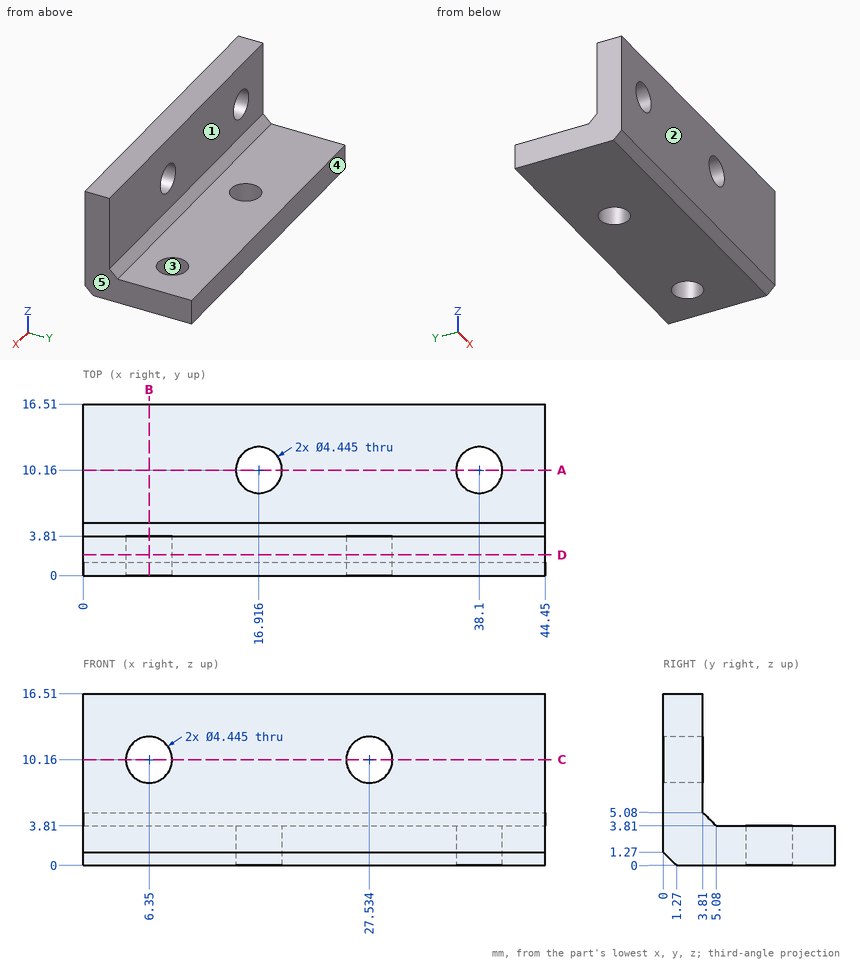
Geometry: see drawing. Coordinates: mm, zero at the bounding-box minimum. A direction names the side the tool comes from. Round coordinates to 2 decimals unless told otherwise and drop trailing zeros. Order: outer loops, then holes, each group sorted by start corner. A loop starts at its lowest first (then second) coordinate and runs counter-clockwise, first axis right, second up. Notation, with made-up numbers: (12, -22) - (63, -22) arc R22 cw to (63, 2) - close; hole circle Ø2 at (-2, 78). An arc over 180 degrees is marked (long way). One line per question, with ' | ' between items. Start each with the question number.
1) Cut plane B-B, the plane x = 6.35. Return the cut outline in (y, z).
2) Contact query for flat-ended pins moving along their axis: P1, Ø8, axis at y = 5.5, z = 9.5, coming from the -X side; P2, Ø3.5, axis at x = 19.5, y = 8, coming from the +Z side; P3, Ø2, axis at x = 25, z = 11.5, coming from the +Y side; P4, Ø2, axis at x = 13.5, y = 6, coming from the +Z side. Output: stop coordinate, or through.
3) Cut plane A-A, the plane y = 10.16. Return the cut outline in (x, z).
4) Cut plane C-C, the plane z = 10.16. Return the cut outline in (x, y).
5) Cut plane D-D, the plane y = 2. Give the number of separate pieces and of enclosed holes in the cut face, then the cut area to 3 significant figures.
6) Ray query, probe 1 along Z at (x, y) = (6.35, 2); probe 2 along Y at (x, z) = (33, 11.75). Return the intervals inside material, ascending.
7) Set-up query: the marked faces 1 and 2. Return all of +Z, -Z, +X, -X, +Y, -Y with unobstructed straight access to the full face (end or side cutting, diameter ignored); none if empty.
8) Pull-direction query (X, two-part tool) for the marked faces 3, 4 and 5; classes: +X half, -X half, draft (parallel to the pull), parting line (faces both ways), or undercut.
Worked out:
1) outline: (0, 1.27) - (1.27, 0) - (16.51, 0) - (16.51, 3.81) - (5.08, 3.81) - (3.81, 5.08) - (3.81, 7.94) - (0, 7.94) - close; (0, 12.38) - (3.81, 12.38) - (3.81, 16.51) - (0, 16.51) - close
2) P1: stops at x = 0 | P2: stops at z = 3.81 | P3: stops at y = 3.81 | P4: stops at z = 3.89
3) outline: (0, 0) - (14.69, 0) - (14.69, 3.81) - (0, 3.81) - close; (19.14, 0) - (35.88, 0) - (35.88, 3.81) - (19.14, 3.81) - close; (40.32, 0) - (44.45, 0) - (44.45, 3.81) - (40.32, 3.81) - close
4) outline: (0, 0) - (4.13, 0) - (4.13, 3.81) - (0, 3.81) - close; (8.57, 0) - (25.31, 0) - (25.31, 3.81) - (8.57, 3.81) - close; (29.76, 0) - (44.45, 0) - (44.45, 3.81) - (29.76, 3.81) - close
5) separate pieces: 1 | enclosed holes: 2 | area: 703 mm^2
6) probe 1: z = 0 to 7.94, 12.38 to 16.51 | probe 2: y = 0 to 3.81
7) face 1: +Z, +X, -X, +Y | face 2: +Z, -Z, +X, -X, -Y
8) face 3: undercut | face 4: draft | face 5: +X half
